```python
from build123d import *

# Parameters (mm, degrees)
SKETCH2_R          = 6.9453125
EXTRUDE1_DEPTH     = 15.10284
EXTRUDE1_TAPER     = 1.783333333
SKETCH11_R         = 6.9453125
EXTRUDE4_DEPTH     = 3.94716
SKETCH13_R         = 6.598046875
EXTRUDE5_DEPTH     = 1.058333333
CIRPATTERN1_COUNT  = 2
SKETCH5_R          = 4.6228
CUT_EXTRUDE3_DEPTH = 40.345708049


with BuildPart() as part:
    # Sketch2 → Extrude1 (new body)
    with BuildSketch(Plane(origin=(3.94716, 0, 0), x_dir=(0, 0, -1), z_dir=(1, 0, 0))):
        Circle(SKETCH2_R)
    extrude(amount=EXTRUDE1_DEPTH, taper=EXTRUDE1_TAPER)



with BuildPart() as body_2:
    # Sketch11 → Extrude4 (new body)
    with BuildSketch(Plane.ZY.offset(-3.94716)):
        Circle(SKETCH11_R)
    extrude(amount=EXTRUDE4_DEPTH)


with BuildPart() as part_1:
    add(part.part)

    add(body_2.part)  # Extrude5 merges body 2
    # Sketch13 → Extrude5 (add)
    with BuildSketch(Plane.ZY.offset(-3.94716)):
        Circle(SKETCH13_R)
    extrude(amount=EXTRUDE5_DEPTH)


with BuildPart() as cirpattern1_1:
    # CirPattern1: pattern copy
    add(part_1.part.rotate(Axis((0, 27.182238006, 0), (0, -1, 0)), 1 * 360 / CIRPATTERN1_COUNT))


with BuildPart() as part_2:
    add(part_1.part)

    # Combine1: union CirPattern1_1
    add(cirpattern1_1.part)

    # Sketch5 → Cut-Extrude3 (cut, through all)
    with BuildSketch(Plane(origin=(19.05, 0, 0), x_dir=(0, 0, -1), z_dir=(1, 0, 0))):
        Circle(SKETCH5_R)
    extrude(amount=-CUT_EXTRUDE3_DEPTH, mode=Mode.SUBTRACT)


solid = part_2.part
```
Source: CAD feature listing. Evaluate the final solid. Frame: model axes, mm. A direction names the side the tool comes from. Round coordinates to 2 decimals unless told otherwise and drop trailing zeros. Loops run counter-clockwise (first coordinate to the right, second up) from the corner with the lowest first, then second, coordinate; pieces in that order, holes last. Notation, with made-up numbers: M 71.25,33.25 L 90.25,33.25 A19 ccw 90.25,46.25 Z; hole C 68,43.5 d2. An arc over 180 degrees is marked long. Use a Markdown table: item, result. Add a question column.
1. Contact query for flat-ended pins moving along their axis: pin 1 (5 mm diameter, centred on x = 14.5, y = -5, fed in from +Z); pin 2 (1 mm diameter, centred on x = 13.5, y = -2, fed in from -Z); pin 3 (3 mm diameter, centred on x = 9.5, z = -4.5, fed in from -Y); pin 4 (8 mm diameter, centred on x = -2, y = 1, fed in from +Z). Output: stop coordinate, or through.
2. Set-up query: faces 4 (the flat face through (-19.05, -4, 3)), 5 (the conical face through (-11.6, -6.55, -1.45)), 6 (the conical face through (11.6, -6.55, 1.45)). Return all of +Z, -Z, +X, -X, +Y, -Y with unobstructed straight access to the full face (end or side cutting, diameter ignored); none if empty.
3. Pull-direction query (Z, two-part tool) for faces 1 (the cylindrical face through (0.27, -2.81, 3.67)), 2 (the cylindrical face through (-0.06, 6.93, -0.46)), 3 (the flat face through (19.05, -3, -4)); classes: +Z half, -Z half, draft (parallel to the pull), parting line (faces both ways), or undercut.
4. Ray query, line 1 along Y through (x, z) = (-3, 0); line 2 along Z through (x, y) = (-4, -4.25); line 3 along Y through (x, z) = (17.5, -2.25). Return the intervals inside material, ascending. Write a range as [from, to].
5. Cut plane C-C, the plane x = -9. Output: boundary loops of the cut face in (y, z).
6. Cut plane B-B, the plane x = 14. Output: boundary loops of the cut face in (y, z), and give its area (3 significant figures).
7. Cut plane A-A, the plane z = 0. Output: boundary loops of the cut face in (x, y).
Solution:
| question | item | result |
|---|---|---|
| 1 | pin 1 | stops at z = 6.13 |
| 1 | pin 2 | stops at z = -6.48 |
| 1 | pin 3 | stops at y = -6.07 |
| 1 | pin 4 | stops at z = 6.95 |
| 2 | face 4 | +Z, -Z, -X, +Y, -Y |
| 2 | face 5 | -X |
| 2 | face 6 | +X |
| 3 | face 1 | undercut |
| 3 | face 2 | parting line |
| 3 | face 3 | draft |
| 4 | line 1 | y = [-6.95, -4.62], [4.62, 6.95] |
| 4 | line 2 | z = [-5.49, -1.82], [1.82, 5.49] |
| 4 | line 3 | y = [-6.12, -4.04], [4.04, 6.12] |
| 5 | outline | C 0,0 d13.58; hole C 0,0 d9.25 |
| 6 | outline | C 0,0 d13.26; hole C 0,0 d9.25 |
| 6 | area | 71.1 mm2 |
| 7 | outline | M -19.05,-6.48 L -3.95,-6.95 L 3.95,-6.95 L 19.05,-6.48 L 19.05,-4.62 L -19.05,-4.62 Z; M -19.05,4.62 L 19.05,4.62 L 19.05,6.48 L 3.95,6.95 L -3.95,6.95 L -19.05,6.48 Z |
